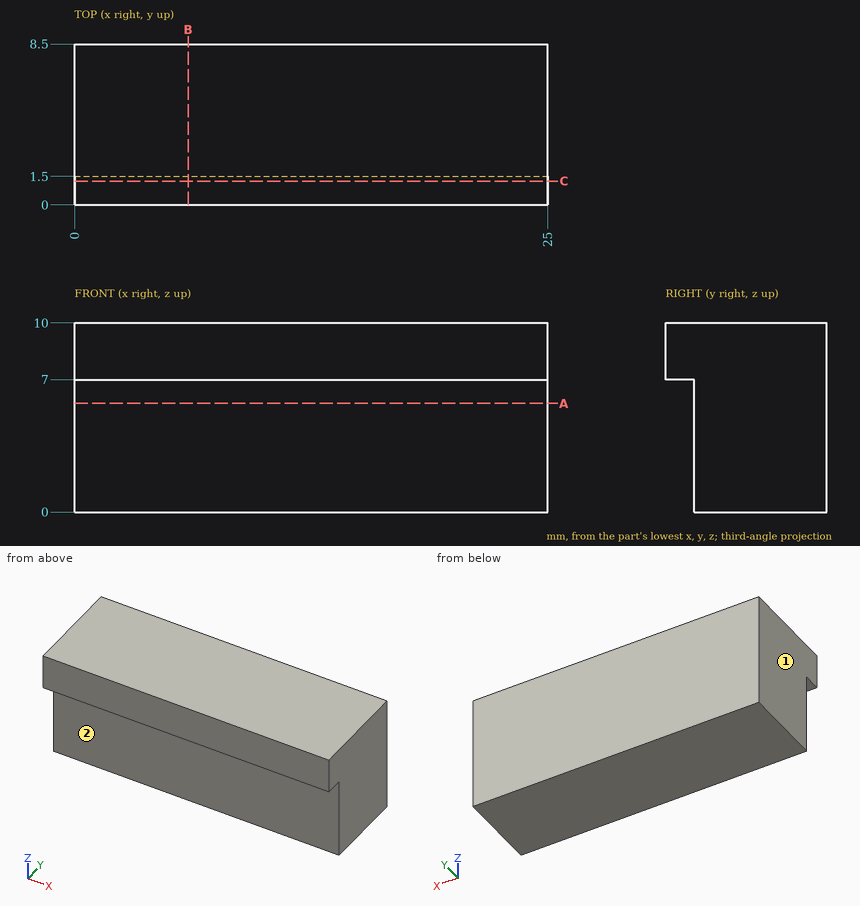
Part print with two shaded views. Sizes in mm from the minimum x, y, z corner. A direction names the side the tool comes from. Round coordinates to 2 decimals unless told otherwise and drop trailing zeros. Write each loop counter-clockwise with the first axis right and the second up, starting at its lowest first coordinate (ties: lowest second). Pieces come first, ordered by that corner, then holes. Notation, with made-up numbers: M 21.25,-29.5 L 68.25,-29.5 A14 ccw 68.25,-13.5 Z; hole C 13,-16 d4. An arc over 180 degrees is marked long. Put each result on its own line as item: value. Start each with the question number.
1) Pin check, flat tips, straight feed: pin 1 Ø2 at (x, z) = (5.5, 3) entering from -Y; pin 2 Ø1.7 at (x, y) = (9.5, 0.5) entering from -Z. Stop position of each tip, or through.
2) Saw through at B-B, the plane x = 6. Write the cut outline in (y, z).
3) 3-axis set-ups, long thin cutter, end or side, ignore diameter. For the marked faces 1 and 2: which of +Z, -Z, +X, -X, +Y, -Y reach the whole face in a straight line?
4) Drill centre line: probe 1 along Y at (x, z) = (17, 3.5). Where is it in solid material? Low to high. Write a range as [from, to].
5) Saw through at A-A, the plane z = 5.75. Write the cut outline in (x, y), and give its area (3 significant figures).
6) Saw through at C-C, the plane y = 1.25. Write the cut outline in (x, z), and give its area (3 significant figures).
Resolved:
1. pin 1: y = 1.5
1. pin 2: z = 7
2. outline: M 0,7 L 1.5,7 L 1.5,0 L 8.5,0 L 8.5,10 L 0,10 Z
3. face 1: +Z, -Z, -X, +Y, -Y
3. face 2: -Z, +X, -X, -Y
4. probe 1: [1.5, 8.5]
5. outline: M 0,1.5 L 25,1.5 L 25,8.5 L 0,8.5 Z
5. area: 175 mm²
6. outline: M 0,7 L 25,7 L 25,10 L 0,10 Z
6. area: 75.0 mm²
